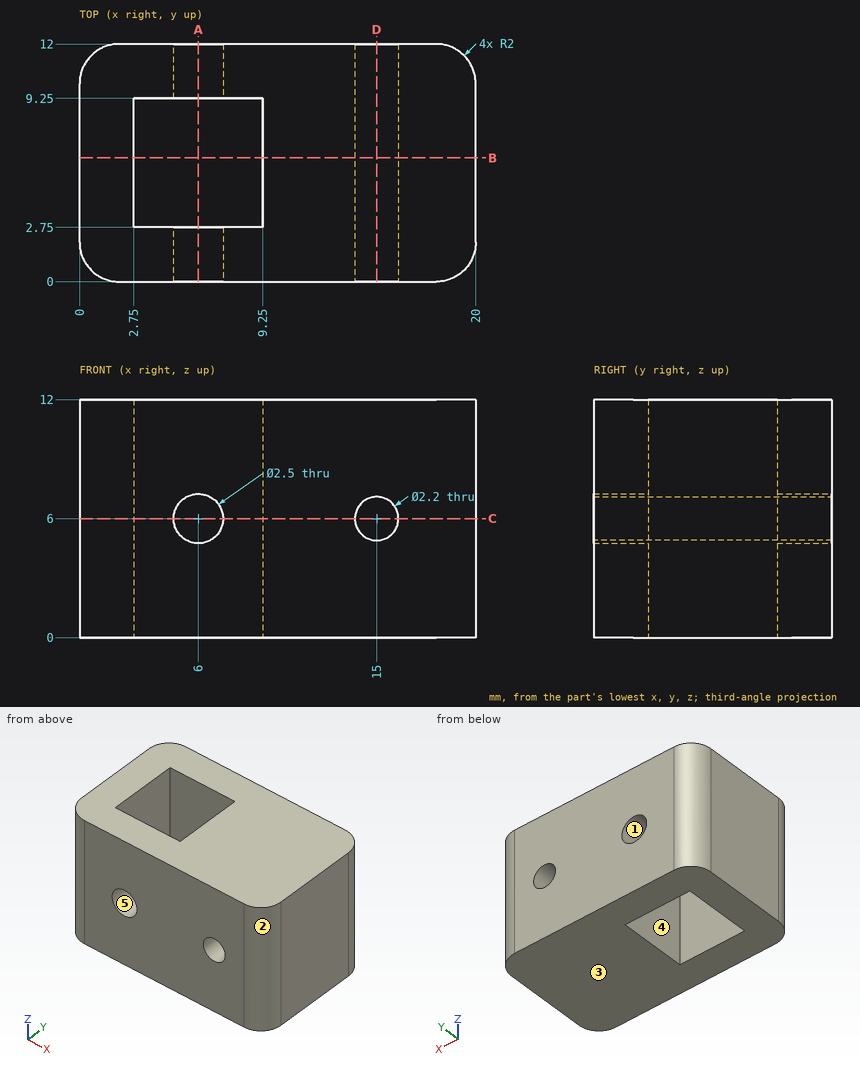
The drawing under review shows one solid part. Ordinate dimensions are in mm from its lowest x, y, z. A direction names the side the tool comes from. Coordinates: 2 decimals unless noted, no trailing zeros. Loops run counter-clockwise (first coordinate to the right, second up) from the corner with the lowest first, then second, coordinate; pieces in that order, holes last. Notation, with made-up numbers: (-26, 50) - (-12, 50) arc R10 cw to (-12, 69) - close; hole circle Ø3 at (2, 25.5). An arc over 180 degrees is marked (long way). Return JSON: item names as keys, results as strings.
Item 1: Take a section at A-A (x = 6). Give the boundary of the cut face in (y, z).
Determined:
{"outline": "(0, 0) - (2.75, 0) - (2.75, 4.75) - (0, 4.75) - close; (0, 7.25) - (2.75, 7.25) - (2.75, 12) - (0, 12) - close; (9.25, 0) - (12, 0) - (12, 4.75) - (9.25, 4.75) - close; (9.25, 7.25) - (12, 7.25) - (12, 12) - (9.25, 12) - close"}
Item 2: Take a section at C-C (z = 6). Give the boundary of the cut face in (x, y).
Determined:
{"outline": "(0, 2) arc R2 ccw to (2, 0) - (4.75, 0) - (4.75, 2.75) - (2.75, 2.75) - (2.75, 9.25) - (4.75, 9.25) - (4.75, 12) - (2, 12) arc R2 ccw to (0, 10) - close; (7.25, 0) - (13.9, 0) - (13.9, 12) - (7.25, 12) - (7.25, 9.25) - (9.25, 9.25) - (9.25, 2.75) - (7.25, 2.75) - close; (16.1, 0) - (18, 0) arc R2 ccw to (20, 2) - (20, 10) arc R2 ccw to (18, 12) - (16.1, 12) - close"}
Item 3: Take a section at B-B (y = 6.25). Give the boundary of the cut face in (x, z), then the cut area to 3 significant figures.
Determined:
{"outline": "(0, 0) - (2.75, 0) - (2.75, 12) - (0, 12) - close; (9.25, 0) - (20, 0) - (20, 12) - (9.25, 12) - close; hole circle Ø2.2 at (15, 6)", "area": "158 mm2"}
Item 4: Take a section at D-D (x = 15). Give the boundary of the cut face in (y, z), then the cut area to 3 significant figures.
Determined:
{"outline": "(0, 0) - (12, 0) - (12, 4.9) - (0, 4.9) - close; (0, 7.1) - (12, 7.1) - (12, 12) - (0, 12) - close", "area": "118 mm2"}
Item 5: For line 1 (X direction, y = 1.95, z = 6); line 2 (X direction, y = 7.5, z = 6); line 3 (Z direction, x = 6, y = 9.9), list the stretches that pass through material, from the lowest coordinate up.
Determined:
{"line 1": "x = 0 to 4.75, 7.25 to 13.9, 16.1 to 20", "line 2": "x = 0 to 2.75, 9.25 to 13.9, 16.1 to 20", "line 3": "z = 0 to 4.75, 7.25 to 12"}
Item 6: Insertion check: pin 1 (2 mm diameter, centred on x = 16, z = 1.5, fed in from -Y). The pin has a flat end and moves straight along its axis. Give the tip position at first contact, or say it passes through.
Determined:
{"pin 1": "stops at y = 0"}
Item 7: For the marked faces 4 and 5, list the 3-axis set-ups (+Z, -Z, +X, -X, +Y, -Y) from which the entire face can be reached by the end or side of a thin tool; tool diameter is ignored.
Determined:
{"face 4": "+Z, -Z", "face 5": "+Y, -Y"}
Item 8: Mouldability with a two-part tool opening along Z and no side actions: class the marked faces 1, 2 and 3 as pulls with the +Z half, pulls with the -Z half, needs draft (parallel to the pull), parting line crosses it, or undercut.
Determined:
{"face 1": "undercut", "face 2": "needs draft", "face 3": "pulls with the -Z half"}
